Geometry: final body of the model. Coordinates: model frame, mm. A direction names the side the tool comes from. Round coordinates to 2 decimals unless told otherwise and drop trailing zeros. Write each loop counter-clockwise with the first axis right and the second up, starting at its lowest first coordinate (ties: lowest second). Pieces come first, ordered by that corner, then holes. Notation, with made-up numbers: M 34.5,76.25 L 46.5,76.25 A22 ccw 46.5,110.25 Z; hole C 80,55 d6. An arc over 180 degrees is marked long. Put each result on its own line as item: value. Start each with the question number.
```python
from build123d import *

# Parameters (mm, degrees)
SKETCH1_W                       = 46
SKETCH1_H                       = 32
SKETCH1_R                       = 3
BOSS_EXTRUDE1_DEPTH             = 22.3
SKETCH3_R                       = 3.8
SKETCH3_R_2                     = 6.6
BOSS_EXTRUDE3_DEPTH             = 2
SKETCH4_R                       = 3
CUT_EXTRUDE1_DEPTH              = 3
SKETCH2_R                       = 12.1
BOSS_EXTRUDE2_DEPTH             = 30.8
CHAMFER1_SIZE                   = 1.4
CHAMFER1_SIZE2                  = 5.224871131
CHAMFER1_PART_2_SIZE            = 1.4
CHAMFER1_PART_2_SIZE2           = 5.224871131
CHAMFER1_PART_3_SIZE            = 1.4
CHAMFER1_PART_3_SIZE2           = 5.224871131
TAP_DRILL_FOR_M3X0_5_TAP1_D     = 2.5
TAP_DRILL_FOR_M3X0_5_TAP1_DEPTH = 2.6
TAP_DRILL_FOR_M3X0_5_TAP1_TIP   = 0.751075774
SKETCH8_R                       = 11.8
CUT_EXTRUDE2_DEPTH              = 0.8
SKETCH7_R                       = 3.2
BOSS_EXTRUDE5_DEPTH             = 2.7


with BuildPart() as part:
    # Sketch1 → Boss-Extrude1 (new body)
    with BuildSketch(Plane(origin=(0, 0, 0), x_dir=(1, 0, 0), z_dir=(0, 1, 0))):
        Rectangle(SKETCH1_W, SKETCH1_H)
        with Locations((7.460620525, 0)):
            Circle(SKETCH1_R, mode=Mode.SUBTRACT)
    extrude(amount=BOSS_EXTRUDE1_DEPTH)

    # Sketch3 → Boss-Extrude3 (add)
    with BuildSketch(Plane(origin=(0, 22.3, 0), x_dir=(1, 0, 0), z_dir=(0, 1, 0))):
        with Locations((-16, -9)):
            Circle(SKETCH3_R)
        with Locations((7.460620525, 0)):
            Circle(SKETCH3_R_2)
        with Locations((17, -9)):
            Circle(SKETCH3_R)
        with Locations((17, 9)):
            Circle(SKETCH3_R)
        with Locations((-16, 9)):
            Circle(SKETCH3_R)
        with BuildLine():
            Line((-8.139379475, -4.95), (-8.139379475, 4.95))
            ThreePointArc((-8.139379475, 4.95), (-5.139379475, 7.95), (-2.139379475, 4.95))
            Line((-2.139379475, 4.95), (-2.139379475, -4.95))
            ThreePointArc((-2.139379475, -4.95), (-5.139379475, -7.95), (-8.139379475, -4.95))
        make_face()
    extrude(amount=BOSS_EXTRUDE3_DEPTH)

    # Sketch4 → Cut-Extrude1 (cut, through all)
    with BuildSketch(Plane.XZ.offset(-22.3)):
        with Locations((7.460620525, 0)):
            Circle(SKETCH4_R)
    extrude(amount=-CUT_EXTRUDE1_DEPTH, mode=Mode.SUBTRACT)

    # Sketch2 → Boss-Extrude2 (add)
    with BuildSketch(Plane.ZY.offset(23)):
        with Locations((2.9, 9.2)):
            Circle(SKETCH2_R)
    extrude(amount=BOSS_EXTRUDE2_DEPTH)

    # Chamfer1
    chamfer1_edges = [part.edges().sort_by_distance(p)[0] for p in [
        (0, 0, -16),
    ]]
    chamfer1_side = [part.faces().sort_by_distance(p)[0] for p in [
        (0, 11.15, -16),
    ]]
    chamfer(chamfer1_edges, length=CHAMFER1_SIZE, length2=CHAMFER1_SIZE2, reference=chamfer1_side[0])

    # Chamfer1 part 2
    chamfer1_part_2_edges = [part.edges().sort_by_distance(p)[0] for p in [
        (23, 0, 0),
    ]]
    chamfer1_part_2_side = [part.faces().sort_by_distance(p)[0] for p in [
        (23, 11.15, 0),
    ]]
    chamfer(chamfer1_part_2_edges, length=CHAMFER1_PART_2_SIZE, length2=CHAMFER1_PART_2_SIZE2, reference=chamfer1_part_2_side[0])

    # Chamfer1 part 3
    chamfer1_part_3_edges = [part.edges().sort_by_distance(p)[0] for p in [
        (0, 0, 16),
    ]]
    chamfer1_part_3_side = [part.faces().sort_by_distance(p)[0] for p in [
        (0, 11.15, 16),
    ]]
    chamfer(chamfer1_part_3_edges, length=CHAMFER1_PART_3_SIZE, length2=CHAMFER1_PART_3_SIZE2, reference=chamfer1_part_3_side[0])

    # Tap Drill for M3x0.5 Tap1
    with Locations(Plane(origin=(0, 24.3, 0), x_dir=(1, 0, 0), z_dir=(0, 1, 0))):
        with Locations((-16, -9), (-16, 9), (17, 9), (17, -9)):
            Hole(TAP_DRILL_FOR_M3X0_5_TAP1_D / 2, depth=TAP_DRILL_FOR_M3X0_5_TAP1_DEPTH)
            with Locations((0, 0, -(TAP_DRILL_FOR_M3X0_5_TAP1_DEPTH + TAP_DRILL_FOR_M3X0_5_TAP1_TIP / 2))):  # 118° drill point
                Cone(0, TAP_DRILL_FOR_M3X0_5_TAP1_D / 2, TAP_DRILL_FOR_M3X0_5_TAP1_TIP, mode=Mode.SUBTRACT)

    # Sketch8 → Cut-Extrude2 (cut)
    with BuildSketch(Plane.ZY.offset(53.8)):
        with Locations((2.9, 9.2)):
            Circle(SKETCH8_R)
    extrude(amount=-CUT_EXTRUDE2_DEPTH, mode=Mode.SUBTRACT)

    # Sketch7 → Boss-Extrude5 (add)
    with BuildSketch(Plane.ZY.offset(53)):
        with Locations((2.9, 9.2)):
            Circle(SKETCH7_R)
    extrude(amount=BOSS_EXTRUDE5_DEPTH)


solid = part.part
```
1) Section B-B, the plane x = 3. Output: boundary loops of the cut face in (y, z).
2) Ray query, probe 1 along Z at (x, y) = (17, 22.6); probe 2 along X at (y, z) = (23.7, 9); probe 3 along Y at (x, z) = (7.5, 6). Return the intervals inside material, ascending.
3) First-contact query: pin 1 (2 mm diameter, centred on y = 23.5, z = -0.5, fed in from +X); pin 2 (2 mm diameter, centred on x = -37.5, y = 7.5, fed in from +Z); pin 3 (6.5 mm diameter, centred on y = 15, z = 2.5, fed in from -X); pin 4 (2 mm diameter, centred on x = 17, z = 9, fed in from -Y). Flat tips, straight axial feed; report the tip coordinate or a pass-through.
4) Draft query along X for faces 1 (the face through (0, 12, -16)), 2 (the face through (-8.139, 23, 0)), 3 (the face through (-5.21, 23.29, -7.95)). Return one class per face: +X half, -X half, draft (parallel to the pull), parting line (faces both ways), or undercut.
5) Access query for faces 4 (the face through (-53.41, 19.15, 9.24)), 5 (the face through (0.867, 23.286, -0.29)), 6 (the face through (-17, 24.3, 8)). Directions: +Z, -Z, +X, -X, +Y, -Y. A direction counts if a zero-diameter tool reaches every point of the face in a straight line with its end or side. Return the directions, or none.
6) Section D-D, the plane x = -29.5. Output: boundary loops of the cut face in (y, z).
7) Section C-C, the plane y = 3.25. Output: boundary loops of the cut face in (x, z), and give its area (3 significant figures).
8) Section A-A, the plane y = 14.75. Output: boundary loops of the cut face in (x, z), and give its area (3 significant figures).
Solved:
1. outline: M 0,-10.78 L 1.4,-16 L 22.3,-16 L 22.3,-4.86 L 24.3,-4.86 L 24.3,4.86 L 22.3,4.86 L 22.3,16 L 1.4,16 L 0,10.78 Z
2. probe 1: z = -12.8 to -10.25, -7.75 to -5.2, 5.2 to 7.75, 10.25 to 12.8
2. probe 2: x = -19.8 to -17.25, -14.75 to -12.2, 13.2 to 15.75, 18.25 to 20.8
2. probe 3: y = 0 to 24.3
3. pin 1: stops at x = 14.06
3. pin 2: stops at z = 14.98
3. pin 3: stops at x = -55.7
3. pin 4: stops at y = 0
4. face 1: draft
4. face 2: -X half
4. face 3: undercut
5. face 4: -X
5. face 5: +Y
5. face 6: +Z, -Z, +X, -X, +Y
6. outline: C 9.2,2.9 d24.2
7. outline: M -53.8,-7.64 L -23,-7.64 L -23,-16 L 23,-16 L 23,16 L -23,16 L -23,13.44 L -53.8,13.44 L -53.8,13.09 L -53,13.09 L -53,-7.29 L -53.8,-7.29 Z; hole C 7.46,0 d6
7. area: 2,080 mm2
8. outline: M -53.8,-7.85 L -23,-7.85 L -23,-16 L 23,-16 L 23,16 L -23,16 L -23,13.65 L -53.8,13.65 L -53.8,13.31 L -53,13.31 L -53,-7.51 L -53.8,-7.51 Z; hole C 7.46,0 d6
8. area: 2,090 mm2
